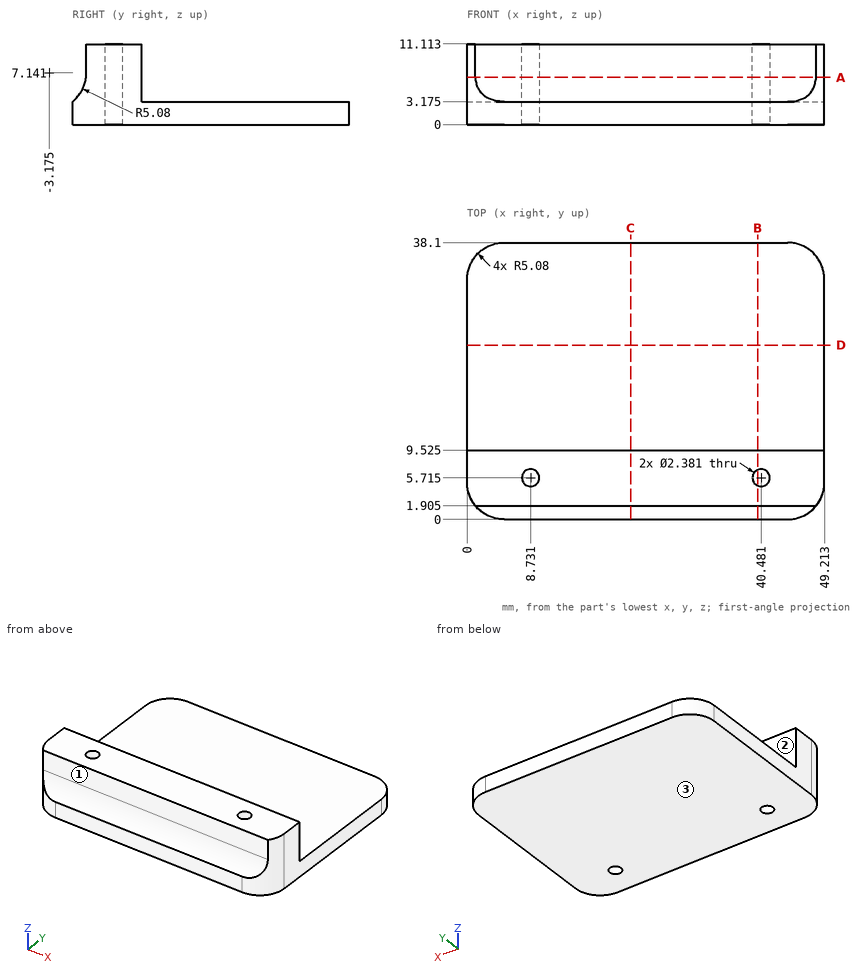
Could you check a few things on this drawing? It's one solid part, dimensions in mm from its lowest x, y, z. A direction names the side the tool comes from. Round coordinates to 2 decimals unless told otherwise and drop trailing zeros. Order: outer loops, then holes, each group sorted by start corner. A loop starts at its lowest first (then second) coordinate and runs counter-clockwise, first axis right, second up. Notation, with made-up numbers: M 66,-23 L 72,-23 A11 cw 72,-17 Z; hole C -23,-12.5 d10. An arc over 180 degrees is marked long. One line per question, with ' | ' between items.
1) Imagine slicing it at A-A, the plane z = 6.5. Write out the boundary of the cut face in (x, y) (1 decimal).
Checked values:
outline: M 0,5.1 A5.1 ccw 1.1,1.9 L 48.1,1.9 A5.1 ccw 49.2,5.1 L 49.2,9.5 L 0,9.5 Z; hole C 8.7,5.7 d2.4; hole C 40.5,5.7 d2.4
2) I need wall thicknesses on line 1 (X direction, y = 6.5, z = 5.5) (1 decimal); line 2 (Y direction, x = 40.5, z = 7.25) (1 decimal); line 3 (X direction, y = 6, z = 5.75) (1 decimal). Which ranges of each line are inside material? Lowest first, please.
Checked values:
line 1: x = 0 to 7.8, 9.6 to 39.6, 41.4 to 49.2 | line 2: y = 1.9 to 4.5, 6.9 to 9.5 | line 3: x = 0 to 7.6, 9.9 to 39.3, 41.6 to 49.2
3) Imagine slicing it at D-D, the plane y = 24. Write out the boundary of the cut face in (x, z) (1 decimal), plus the area to 3 significant figures.
Checked values:
outline: M 0,0 L 49.2,0 L 49.2,3.2 L 0,3.2 Z | area: 156 mm²
4) On a 3-axis mill with a long thin cutter (end or side, diameter ignored), from which of +Z, -Z, +X, -X, +Y, -Y can I reach the whole of each face in a straight line? I mean the marked faces 1, 2 and 3. Say none if no direction works.
Checked values:
face 1: +Z, +X, -X, -Y | face 2: +Z, +X, -X, +Y | face 3: -Z, +X, -X, +Y, -Y
5) I'm going to push flat-ended pins straight in: pin 1 Ø3 at (x, z) = (26.5, 9.5) entering from -Y (1 decimal); pin 2 Ø1 at (y, z) = (10.5, 4.5) entering from -X; pin 3 Ø4 at (x, y) = (24, 27.5) entering from +Z (1 decimal); pin 4 Ø6 at (x, z) = (26, 6.5) entering from +Y (1 decimal). Where does each tip first touch, or does it pass through?
Checked values:
pin 1: stops at y = 1.9 | pin 2: passes through | pin 3: stops at z = 3.2 | pin 4: stops at y = 9.5
6) Imagine slicing it at C-C, the plane x = 22.5. Write out the boundary of the cut face in (y, z) (1 decimal), plus the area to 3 significant figures.
Checked values:
outline: M 0,0 L 38.1,0 L 38.1,3.2 L 9.5,3.2 L 9.5,11.1 L 1.9,11.1 L 1.9,7.1 A5.1 cw 0,3.2 Z | area: 184 mm²
7) Imagine slicing it at B-B, the plane x = 40. Write out the boundary of the cut face in (y, z) (1 decimal).
Checked values:
outline: M 0,0 L 4.6,0 L 4.6,11.1 L 1.9,11.1 L 1.9,7.1 A5.1 cw 0,3.2 Z; M 6.8,0 L 38.1,0 L 38.1,3.2 L 9.5,3.2 L 9.5,11.1 L 6.8,11.1 Z
